Part model, mm, in its own coordinate system. A direction names the side the tool comes from. Give positions to 0.01 mm unless a question says otherwise; leave off trailing zeros. Order: outer loops, then holes, each group sorted by start corner. A loop starts at its lowest first (then second) coordinate and runs counter-clockwise, first axis right, second up. Notation, with made-up numbers: (4, 87) - (29, 87) arc R15 cw to (29, 105) - close; hole circle Ø3 at (-28.75, -0.5). An arc over 180 degrees is marked (long way). Use one line per item in the form item = value. Start each with the question number.
1. Pin check, flat tips, straight feed: P1, Ø1.5, axis at x = 9.5, z = -21, coming from the -Y side; P2, Ø3, axis at y = -14.5, z = -25, coming from the -X side; P3, Ø2, axis at x = -16.5, z = -27.5, coming from the -Y side. Stop position of each tip, or through.
2. Pull direction Z, two halves, no side cores. Call faces 4 (the face through (-1.5, -11, -24)), 5 (the face through (17.824, -0.507, -28.39)), 6 (the face through (-14.05, -0.74, -26.68)), 7 (the face through (-1.365, 9.298, -24.998)): +Z half, -Z half, draft (parallel to the pull), parting line (faces both ways), or undercut.
3. Band-saw the part on B-B, the plane y = -2.5. List the corners of the cut face in (x, z).
4. Band-saw the part on A-A, the plane z = -21.25. State how many separate pieces and enclosed holes the cut face has, plus the area to 3 significant figures.
5. Tool access for faces 1 (the face through (-11.77, -1.14, -22.54)), 2 (the face through (11.77, 1.14, -22.54)), 3 (the face through (10, 1.5, -23)): list every direction of +Z, -Z, +X, -X, +Y, -Y with a clear straight run to the whole face (end or side of a thin tool).
6. Drill centre lines: line 1 (X direction, y = -13.5, z = -26.25); line 2 (Z direction, x = -0.25, y = -16); line 3 (X direction, y = 15.5, z = -29). Where is each one in solid material? Low to high.
from build123d import *

# Parameters (mm, degrees)
F7_DEPTH         = 1.5
F7_COPIES_COUNT  = 4
F8_SIZE          = 0.5
F9_R             = 2.15
F10_DEPTH        = 1.5
F10_COPIES_COUNT = 4
F11_R            = 1
F12_DEPTH        = 3
F12_COPIES_COUNT = 4


# Not quite as in the source:
# - a pattern or mirror of a feature is missing from the dataset's text; its kind, count and spacing are read off the source's solid


with BuildPart() as f1:
    # F0 (on Top) → F1 (revolve)
    with BuildSketch(Plane.XY):
        with BuildLine():
            Line((0, -20), (0, 20))
            ThreePointArc((0, 20), (-20, 0), (0, -20))
        make_face()
    revolve(axis=Axis((0, 0, 0), (0, -1, 0)))

    # F2 (on Front) → F3 (revolve)
    with BuildSketch(Plane.XZ):
        with BuildLine():
            ThreePointArc((-4.5983759881, -20.2777777778), (-5.1275841713, -19.7652786452), (-5.6, -19.2))
            ThreePointArc((-5.6, -19.2), (-7.6082065121, -18.4963562268), (-9.5302879751, -17.5833333333))
            ThreePointArc((-9.5302879751, -17.5833333333), (-7.1916475208, -19.1635939597), (-4.5983759881, -20.2777777778))
        make_face()
        with BuildLine():
            Line((0, -21), (0, -20))
            ThreePointArc((0, -20), (-2.8284271247, -19.7989898732), (-5.6, -19.2))
            ThreePointArc((-5.6, -19.2), (-5.1275841713, -19.7652786452), (-4.5983759881, -20.2777777778))
            ThreePointArc((-4.5983759881, -20.2777777778), (-2.3273733406, -20.8183444869), (0, -21))
        make_face()
        with BuildLine():
            Line((0, -22), (0, -21))
            ThreePointArc((0, -21), (-2.3273733406, -20.8183444869), (-4.5983759881, -20.2777777778))
            ThreePointArc((-4.5983759881, -20.2777777778), (-2.4551533104, -21.5553201464), (0, -22))
        make_face()
    revolve(axis=Axis((0, 0, -21), (0, 0, -1)))

    # F4 (on Top) → F5 (revolve, cut)
    with BuildSketch(Plane.XY):
        with BuildLine():
            ThreePointArc((0, -20), (20, 0), (0, 20))
            Line((0, 20), (0, -20))
        make_face()
    revolve(axis=Axis((0, 0, 0), (0, -1, 0)), mode=Mode.SUBTRACT)

    # F6 (on Front) → F7 (join, symmetric)
    with BuildSketch(Plane.XZ):
        with BuildLine():
            ThreePointArc((16.7667947961, -25.7420411911), (12.0468652107, -22.6201202145), (8.8194778429, -17.9716692195))
            Line((8.8194778429, -17.9716692195), (5.3091861203, -19.8894418917))
            ThreePointArc((5.3091861203, -19.8894418917), (9.3769721823, -25.5877227261), (15.2332052039, -29.4246254756))
            ThreePointArc((15.2332052039, -29.4246254756), (17.8412921423, -28.3501281294), (16.7667947961, -25.7420411911))
        make_face()
    f7 = extrude(amount=F7_DEPTH, both=True)

    # F7_copies: F7 ×4 about axis
    f7_copies_axis = Axis((0, 0, 0), (0, 0, 1))
    for i in range(1, F7_COPIES_COUNT):
        add(f7.rotate(f7_copies_axis, i * 360 / F7_COPIES_COUNT))

    # F8
    f8_edges = [f1.edges().sort_by_distance(p)[0] for p in [
        (9.396954, 1.5, -25.606894),
        (17.841292, 1.5, -28.350128),
        (12.067102, 1.5, -22.639869),
        (12.067102, -1.5, -22.639869),
        (17.841292, -1.5, -28.350128),
        (9.396954, -1.5, -25.606894),
        (-12.067102, 1.5, -22.639869),
        (-12.067102, -1.5, -22.639869),
        (-9.396954, 1.5, -25.606894),
        (-17.841292, 1.5, -28.350128),
        (-9.396954, -1.5, -25.606894),
        (1.5, 9.396954, -25.606894),
        (-1.5, 9.396954, -25.606894),
        (1.5, 12.067102, -22.639869),
        (1.5, 17.841292, -28.350128),
        (-1.5, 12.067102, -22.639869),
        (-1.5, -9.396954, -25.606894),
        (1.5, -9.396954, -25.606894),
        (1.5, -12.067102, -22.639869),
        (-1.5, -12.067102, -22.639869),
        (-1.5, -17.841292, -28.350128),
    ]]
    chamfer(f8_edges, length=F8_SIZE)

    # F9 (on Front) → F10 (cut, through all)
    with BuildSketch(Plane.XZ):
        with Locations((16, -27.5833333333)):
            Circle(F9_R)
    f10 = extrude(amount=-F10_DEPTH, mode=Mode.SUBTRACT)

    # F10_copies: F10 ×4 about axis
    f10_copies_axis = Axis((0, 0, 0), (0, 0, 1))
    for i in range(1, F10_COPIES_COUNT):
        add(f10.rotate(f10_copies_axis, i * 360 / F10_COPIES_COUNT), mode=Mode.SUBTRACT)

    # F11 (on face) → F12 (cut, through all)
    with BuildSketch(Plane.XZ.offset(1.5)):
        with Locations((16, -27.5833333333)):
            Circle(F11_R)
    f12 = extrude(amount=-F12_DEPTH, mode=Mode.SUBTRACT)

    # F12_copies: F12 ×4 about axis
    f12_copies_axis = Axis((0, 0, 0), (0, 0, 1))
    for i in range(1, F12_COPIES_COUNT):
        add(f12.rotate(f12_copies_axis, i * 360 / F12_COPIES_COUNT), mode=Mode.SUBTRACT)


solid = f1.part
From the geometry:
q1.P1 = -1.5
q1.P2 = -1.5
q1.P3 = 0
q2.face_4 = draft
q2.face_5 = parting line
q2.face_6 = undercut
q2.face_7 = -Z half
q3.outline = (-9.2, -17.58) arc R14.79 ccw to (-3.86, -20.28) arc R6.54 ccw to (3.86, -20.28) arc R14.79 ccw to (9.2, -17.58) arc R19.84 cw to start
q4.separate_pieces = 5
q4.enclosed_holes = 0
q4.area = 86.4 mm²
q5.face_1 = -X, -Y
q5.face_2 = +X, +Y
q5.face_3 = -Z, +X, +Y
q6.line_1 = -1.5 to 1.5
q6.line_2 = -29.58 to -28.58, -26.58 to -25.4
q6.line_3 = 0 to 1.49
